Autodesk Inventor part; units mm, degrees
ref_plane "YZ Plane" through (0, 0, 0) normal (1, 0, 0) x (0, 1, 0)
ref_plane "XZ Plane" through (0, 0, 0) normal (0, 1, 0) x (-1, 0, 0)
ref_plane "XY Plane" through (0, 0, 0) normal (0, 0, 1) x (1, 0, 0)
sketch "Эскиз1" plane through (0, 0, 0) normal (0, 1, 0) x (-1, 0, 0)
  line L0 (70.6667, 46) -> (-29.3333, 46)
  line L1 (-29.3333, 46) -> (-29.3333, 19.5)
  line L2 (-29.3333, 19.5) -> (70.6667, 19.5)
  line L3 (70.6667, 19.5) -> (70.6667, 46)
  line L4 (-29.3333, 19.5) -> (-9.3333, 19.5)
  line L5 (-9.3333, 19.5) -> (-9.3333, -5)
  line L6 (-9.3333, -5) -> (-29.3333, -5)
  line L7 (-29.3333, -5) -> (-29.3333, 19.5)
  point P0 (0, 0)
  dimension "d0" = 26.5
  dimension "d1" = 100
  dimension "d2" = 20
  dimension "d5" = 51
extrude "Выдавливание1" add sketch "Эскиз1" along normal blind 290
properties part number "MegaUgolok"
Work out the finished part from the listing and answer in its coordinate system (mm). Round coordinates to 2 decimals unless told otherwise and drop trailing zeros. Loops run counter-clockwise (first coordinate to the right, second up) from the corner with the lowest first, then second, coordinate; pieces in that order, holes last. Notation, with made-up numbers: (35, 85.5) -> (69, 85.5) arc R17 cw to (69, 116.5) -> close; hole circle Ø7 at (88, 84.25). An arc over 180 degrees is marked (long way). Use one line per item in the form item = value.
(1) Find section B-B on x = -14. Give the vertices of the cut face in (y, z), then the cut area to 4 significant figures.
Answer list:
outline = (0, 19.5) -> (290, 19.5) -> (290, 46) -> (0, 46) -> close
area = 7,685 mm2
(2) Find section C-C on z = 2. Give the vertices of the cut face in (x, y), then the cut area to 3 significant figures.
Answer list:
outline = (9.33, 0) -> (29.33, 0) -> (29.33, 290) -> (9.33, 290) -> close
area = 5,800 mm2
(3) For a pull along Z with two mould halves and no side action, classify faces 1 (the flat face through (-30, 143, 19.5)), 2 (the flat face through (9.333, 143, 7)), 3 (the flat face through (-21, 143, 46)) as released by +Z, released by -Z, zero draft, split by the parting line, or undercut.
Answer list:
face_1 = released by -Z
face_2 = zero draft
face_3 = released by +Z
(4) Flat-ended cylindrical pins translate along their axes: P1, Ø8, axis at x = -22, y = 259, coming from the -Z side; P2, Ø8, axis at y = 61, z = 4.5, coming from the -X side; P3, Ø12, axis at x = 1.5, z = 9.5, coming from the +Y side. Find the tip coordinate at first contact, or state that the pin passes through.
Answer list:
P1 = 19.5
P2 = 9.33
P3 = through
(5) Straight lines are drawn through the part: line 1 (X direction, y = 18, z = 8.5); line 2 (Z direction, x = -61, y = 35.5). For each, find the intervals that lie inside material, in ascending order.
Answer list:
line_1 = 9.33 to 29.33
line_2 = 19.5 to 46
(6) Find section A-A on y = 228.5. Give the vertices of the cut face in (x, z).
Answer list:
outline = (-70.67, 19.5) -> (9.33, 19.5) -> (9.33, -5) -> (29.33, -5) -> (29.33, 46) -> (-70.67, 46) -> close
